Here's how the part is built. I have some questions about the finished solid (model axes, mm). A direction names the side the tool comes from. Round coordinates to 2 decimals unless told otherwise and drop trailing zeros. Order: outer loops, then holes, each group sorted by start corner. A loop starts at its lowest first (then second) coordinate and runs counter-clockwise, first axis right, second up. Notation, with made-up numbers: (-21.5, 25) - (12.5, 25) arc R13 ccw to (12.5, 45) - close; hole circle Ø10 at (17.5, 88). An arc over 180 degrees is marked (long way). Answer as a JSON object with one key per item and string values.
```python
from build123d import *

# Parameters (mm, degrees)
SKETCH1_R           = 10
BOSS_EXTRUDE1_DEPTH = 45
SKETCH2_R           = 2.65
CUT_EXTRUDE1_DEPTH  = 48.16990566
SKETCH3_R           = 5
CUT_EXTRUDE2_DEPTH  = 1.5


with BuildPart() as part:
    # Sketch1 → Boss-Extrude1 (new body)
    with BuildSketch(Plane.XY):
        Circle(SKETCH1_R)
    extrude(amount=-BOSS_EXTRUDE1_DEPTH)

    # Sketch2 → Cut-Extrude1 (cut, through all)
    with BuildSketch(Plane.XY):
        Circle(SKETCH2_R)
    extrude(amount=-CUT_EXTRUDE1_DEPTH, mode=Mode.SUBTRACT)

    # Sketch3 → Cut-Extrude2 (cut)
    with BuildSketch(Plane.XY):
        Circle(SKETCH3_R)
    extrude(amount=-CUT_EXTRUDE2_DEPTH, mode=Mode.SUBTRACT)


solid = part.part
```
1. For faces 1 (the face through (-5, -2, 0)), 2 (the face through (-1.08, -4.88, -0.74)), which set-ups out of +Z, -Z, +X, -X, +Y, -Y let a thin tool reach every point of the face, with its end or its side?
Responses:
{"face 1": "+Z, +X, -X, +Y, -Y", "face 2": "+Z"}
2. Thinking about a two-plate mould opening in Y: for faces 3 (the face through (-2.17, -9.76, -22.18)), 4 (the face through (2, -2, -45)), 5 (the face through (2.45, -1.01, -22.95)), which applies, pulls with the +Y half, pulls with the -Y half, needs draft (parallel to the pull), parting line crosses it, or undercut?
Responses:
{"face 3": "parting line crosses it", "face 4": "needs draft", "face 5": "undercut"}
3. Imagine slicing it at A-A (x = 0). List the corners of the cut face in (y, z) for me.
Responses:
{"outline": "(-10, -45) - (-2.65, -45) - (-2.65, -1.5) - (-5, -1.5) - (-5, 0) - (-10, 0) - close; (2.65, -45) - (10, -45) - (10, 0) - (5, 0) - (5, -1.5) - (2.65, -1.5) - close"}
4. If I drill on L1, parallel to Y at x = 0, z = -17; L2, parallel to Y at x = 0, z = -0.45; L3, parallel to Z at x = 4.25, y = 0.75, over which ranges is the centre line in solid material (lowest first)? Write a range as [from, to].
Responses:
{"L1": "[-10, -2.65], [2.65, 10]", "L2": "[-10, -5], [5, 10]", "L3": "[-45, -1.5]"}
5. Imagine slicing it at D-D (z = -41). List the corners of the cut face in (x, y) for me.
Responses:
{"outline": "circle Ø20 at (0, 0); hole circle Ø5.3 at (0, 0)"}
6. Imagine slicing it at C-C (x = 3.25). List the corners of the cut face in (y, z) for me, plus the area to 3 significant figures.
Responses:
{"outline": "(-9.46, -45) - (9.46, -45) - (9.46, 0) - (3.8, 0) - (3.8, -1.5) - (-3.8, -1.5) - (-3.8, 0) - (-9.46, 0) - close", "area": "840 mm2"}
7. For P1, Ø1, axis at x = -5, z = -21.5, coming from the +Y side; P2, Ø12, axis at x = 2, z = -14, coming from the -Y side; P3, Ø5, axis at x = -0.5, y = -1.5, coming from the +Z side; P4, Ø1, axis at x = 5.5, z = -23, coming from the +Y side, each with a flat end and sliding along its axis, tell me the tip position at first contact or that it passes through.
Responses:
{"P1": "y = 8.93", "P2": "y = -10", "P3": "z = -1.5", "P4": "y = 8.66"}
